```python
from build123d import *

# Parameters (mm, degrees)
CORTAR_EXTRUIR1_START = -2.54
CORTAR_EXTRUIR1_DEPTH = 2.54


# Read off the part's stored shape, not the designer's step: Cortar-Extruir1
with BuildPart() as part:
    # Croquis1 → Revolución1 (revolve)
    with BuildSketch(Plane(origin=(0, 0, 0), x_dir=(0, 0, -1), z_dir=(1, 0, 0))):
        Polygon((0, 0), (0, 11.938), (1.778, 11.938), (1.778, 9.525), (15.494, 9.525), (15.494, 19.05), (18.034, 19.05), (18.034, 10.668), (125.984, 10.668), (125.984, 0), align=None)
    revolve(axis=Axis((0, 0, -125.984), (0, 0, 1)))

    # Cortar-Extruir1 outline → Cortar-Extruir1 (cut)
    with BuildSketch(Plane.XY.offset(-15.494).offset(CORTAR_EXTRUIR1_START)):
        with BuildLine():
            Line((-7.156259894, -17.654756989), (-12.7, 0))
            Line((-12.7, 0), (-7.156259894, 17.654756989))
            ThreePointArc((-7.156259894, 17.654756989), (-19.05, 0), (-7.156259894, -17.654756989))
        make_face()
        with BuildLine():
            Line((12.7, 0), (7.156259894, -17.654756989))
            ThreePointArc((7.156259894, -17.654756989), (19.05, 0), (7.156259894, 17.654756989))
            Line((7.156259894, 17.654756989), (12.7, 0))
        make_face()
    extrude(amount=CORTAR_EXTRUIR1_DEPTH, mode=Mode.SUBTRACT)


solid = part.part
```
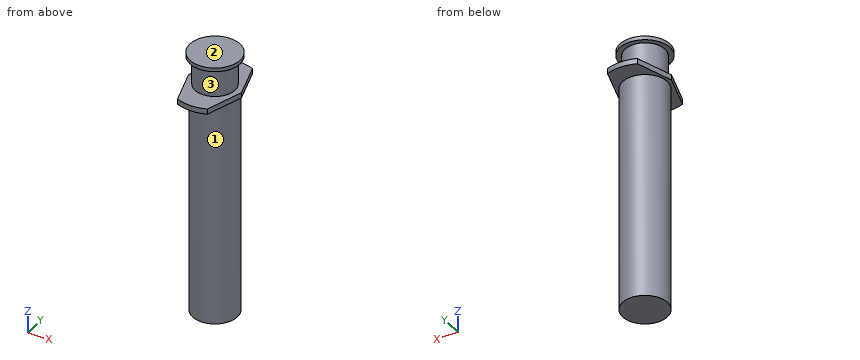
Model file for the job. Use its own axes, mm. Face numbers are marked on the shaded views. A direction names the side the tool comes from. Coordinates: 2 decimals unless noted, no trailing zeros. Loops run counter-clockwise (first coordinate to the right, second up) from the corner with the lowest first, then second, coordinate; pieces in that order, holes last. Notation, with made-up numbers: (61, 23.25) - (105, 23.25) arc R5 cw to (105, 32.25) - close; hole circle Ø2 at (51.25, 26). An arc over 180 degrees is marked (long way). Write item = value, one per line. Start each with the question number.
Item 1: 3-axis set-ups, long thin cutter, end or side, ignore diameter. For the marked faces 1, 2 and 3: which of +Z, -Z, +X, -X, +Y, -Y reach the whole face in a straight line?
Item 2: Saw through at A-A, the plane x = 0. List the corners of the cut face in (y, z) (3 decimals), then the cut area to 3 significant figures.
Item 3: Saw through at D-D, the plane y = 14. List the corners of the cut face in (x, z).
Item 4: Saw through at C-C, the plane z = -8.5. List the corners of the cut face in (x, y) (3 decimals).
Item 5: Saw through at B-B, the plane y = 2.5. List the corners of the cut face in (x, z).
Item 6: Drop flat-ended pins along their axis: pin 1 Ø12 at (y, z) = (12, -14.5) entering from +X; pin 2 Ø8 at (y, z) = (9.5, -15.5) entering from -X; pin 3 Ø1.5 at (x, y) = (-4.5, -12) entering from +Z. Give the stop position or say it passes through.
Item 7: Wall check: probe 1 along Y at (x, z) = (0, -43); probe 2 along Z at (x, y) = (7, 12). Give the ranges that are in metal, low to high. Write a range as [from, to].
Answers:
q1.face_1 = -Z
q1.face_2 = +Z, +X, -X, +Y, -Y
q1.face_3 = none
q2.outline = (-19.05, -18.034) - (-10.668, -18.034) - (-10.668, -125.984) - (10.668, -125.984) - (10.668, -18.034) - (19.05, -18.034) - (19.05, -15.494) - (9.525, -15.494) - (9.525, -1.778) - (11.938, -1.778) - (11.938, 0) - (-11.938, 0) - (-11.938, -1.778) - (-9.525, -1.778) - (-9.525, -15.494) - (-19.05, -15.494) - close
q2.area = 2,700 mm2
q3.outline = (-8.3, -18.03) - (8.3, -18.03) - (8.3, -15.49) - (-8.3, -15.49) - close
q4.outline = circle Ø19.05 at (0, 0)
q5.outline = (-11.91, -18.03) - (-10.37, -18.03) - (-10.37, -125.98) - (10.37, -125.98) - (10.37, -18.03) - (11.91, -18.03) - (11.91, -15.49) - (9.19, -15.49) - (9.19, -1.78) - (11.67, -1.78) - (11.67, 0) - (-11.67, 0) - (-11.67, -1.78) - (-9.19, -1.78) - (-9.19, -15.49) - (-11.91, -15.49) - close
q6.pin_1 = 10.79
q6.pin_2 = -10.97
q6.pin_3 = -15.49
q7.probe_1 = [-10.67, 10.67]
q7.probe_2 = [-18.03, -15.49]
